Verification items for the finished model (mm, model axes). Face numbers are marked on the shaded views. A direction names the side the tool comes from. Coordinates: 2 decimals unless noted, no trailing zeros. Write each loop counter-clockwise with the first axis right and the second up, starting at its lowest first coordinate (ties: lowest second). Pieces come first, ordered by that corner, then holes. Notation, with made-up numbers: (-1, 80) -> (23, 80) arc R13 cw to (23, 91) -> close; hole circle Ø7 at (-9.5, 0.5). An arc over 180 degrees is marked (long way). Use a Markdown table: item, result. Add a question column.
from build123d import *

# Parameters (mm, degrees)
F0_W     = 19.4115899503
F0_H     = 28.2941963524
F1_DEPTH = 25.4
F3_DEPTH = 25.4


with BuildPart() as f1:
    # F0 (on Top) → F1 (new body)
    with BuildSketch(Plane.XY):
        with Locations((-9.7057949752, 14.1470981762)):
            Rectangle(F0_W, F0_H)
    extrude(amount=F1_DEPTH)

    # F2 (on face) → F3 (join)
    with BuildSketch(Plane.XY.offset(25.4)):
        with BuildLine():
            Line((0, 4.6914111863), (0, 21.2403103669))
            ThreePointArc((0, 21.2403103669), (-18.3741405241, 12.9658607766), (0, 4.6914111863))
        make_face()
    extrude(amount=F3_DEPTH)


solid = f1.part
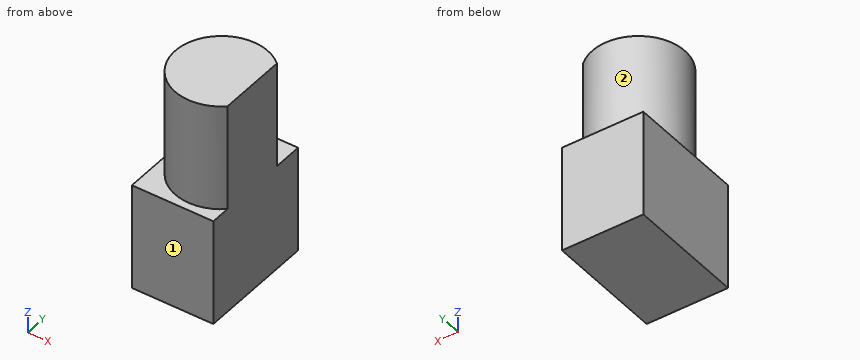
1) Set-up check for the marked faces 1 and 2: record each of +Z, -Z, +X, -X, +Y, -Y from which the full face is reachable in a straight line by a thin tool's end or side.
2) Gauge pin test, flat end, axial feed: pin 1 (1 mm diameter, centred on x = -9, z = 28.5, fed in from +Y). Record the tip position at first contact, or that the pin passes through.
3) Cross-section at B-B on y = 3.75. Record the boundary of the cut face in (x, z).
4) Thickness scan on L1, parallel to X at y = 7.25, z = 36; L2, parallel to X at y = 6.75, z = 48; L3, parallel to Y at x = -10.75, z = 27.5. Record the ranges inside material, lowest first.
5) Cross-section at D-D on z = 44. Record the boundary of the cut face in (x, y).
6) Cross-section at A-A on x = -6. Record the boundary of the cut face in (y, z).
7) Cross-section at C-C on y = 10.5. Record the boundary of the cut face in (x, z).
Returned:
| question | item | result |
|---|---|---|
| 1 | face 1 | +Z, -Z, +X, -X, -Y |
| 1 | face 2 | +Z |
| 2 | pin 1 | stops at y = 23.95 |
| 3 | outline | (-19.41, 0) -> (0, 0) -> (0, 25.4) -> (-1.23, 25.4) -> (-1.23, 50.8) -> (-13.42, 50.8) -> (-13.42, 25.4) -> (-19.41, 25.4) -> close |
| 4 | L1 | x = -16.78 to 0 |
| 4 | L2 | x = -16.46 to 0 |
| 4 | L3 | y = 2.46 to 23.47 |
| 5 | outline | (0, 4.69) -> (0, 21.24) arc R11.05 ccw (long way) to start |
| 6 | outline | (0, 0) -> (28.29, 0) -> (28.29, 25.4) -> (23.94, 25.4) -> (23.94, 50.8) -> (2, 50.8) -> (2, 25.4) -> (0, 25.4) -> close |
| 7 | outline | (-19.41, 0) -> (0, 0) -> (0, 50.8) -> (-18.1, 50.8) -> (-18.1, 25.4) -> (-19.41, 25.4) -> close |
